Could you check a few things on this model? Use its own coordinates, in mm. A direction names the side the tool comes from. Give positions to 0.01 mm unless a question says otherwise; leave off trailing zeros. Order: outer loops, then holes, each group sorted by start corner. A loop starts at its lowest first (then second) coordinate and runs counter-clockwise, first axis right, second up. Notation, with made-up numbers: (11, -2.5) -> (41, -2.5) arc R18 cw to (41, 21.5) -> close; hole circle Ø2 at (66.25, 83.5). An arc over 180 degrees is marked (long way). Answer as CSV lines item,"result". Start each with the question number.
(1) I need wall thicknesses on L1, parallel to Y at x = -12, z = -12.55; L2, parallel to Z at x = -4, y = 2.5; L3, parallel to X at y = 10, z = -13.95. Which ranges of each line are inside material? Lowest first, please.
(2) Will these pins go through, and if not, where does the flat tip stop? pin 1 Ø5 at (x, y) = (13, 11.5) entering from +Z; pin 2 Ø5 at (y, z) = (12.5, 1) entering from -X; pin 3 Ø4.5 at (y, z) = (7.5, -6.5) entering from +X; pin 4 Ø12 at (x, z) = (0.5, -2) entering from -Y.
(3) I want a section at C-C (x = -8). Please give me the cut outline in (y, z).
(4) We'd pull the mould along X, two halves only. Please class faces 4 (the face through (11.231, 12.727, 4.728)), 5 (the face through (1, 20, -6)), 6 (the face through (0, 10, -5)): released by +X, released by -X, zero draft, split by the parting line, or undercut.
(5) I want a section at B-B (y = 10). Please give me the cut outline in (x, z).
(6) On a 3-axis mill with a long thin cutter (end or side, diameter ignored), from which of +Z, -Z, +X, -X, +Y, -Y can I reach the whole of each face in a straight line? I mean faces 1 (the face through (-9, 10, -12)), 2 (the face through (-11.642, 12.727, -13.521)), 3 (the face through (3, 10, -7)). Say none if no direction works.
(7) I want a section at D-D (z = 0.5). Please give me the cut outline in (x, y), plus the area to 3 significant figures.
(8) I want a section at A-A (x = -12). Please give me the cut outline in (y, z).
Autodesk Inventor part; units mm, degrees
ref_plane "YZ Plane" through (0, 0, 0) normal (1, 0, 0) x (0, 1, 0)
ref_plane "XZ Plane" through (0, 0, 0) normal (0, 1, 0) x (-1, 0, 0)
ref_plane "XY Plane" through (0, 0, 0) normal (0, 0, 1) x (1, 0, 0)
sketch "Sketch4" plane through (0, 0, 0) normal (0, 1, 0) x (-1, 0, 0)
  line L0 (0, 0) -> (0, -12)
  line L1 (0, -12) -> (20, -12)
  line L2 (20, -12) -> (0, -12)
  line L3 (0, -12) -> (0, -15)
  line L4 (0, -15) -> (20, -15)
  line L5 (20, -15) -> (20, -12)
  line L6 (0, 0) -> (-15.5885, 9)
  line L7 (0, 0) -> (18, 0) construction
  line L8 (-15.5885, 9) -> (0, 0)
  line L9 (0, 0) -> (-1.5, -2.5981)
  line L10 (-1.5, -2.5981) -> (-17.0885, 6.4019)
  line L11 (-17.0885, 6.4019) -> (-15.5885, 9)
  line L12 (0, 0) -> (0, -15)
  line L13 (0, -15) -> (-3, -15)
  line L14 (-3, -15) -> (-3, 0)
  line L15 (-3, 0) -> (0, 0)
  dimension "d16" = 12
  dimension "d17" = 20
  dimension "d18" = 3
  dimension "d19" = 18
  dimension "d20" = 150
  dimension "d21" = 3
  dimension "d24" = 3
extrude "Extrusion5" add sketch "Sketch4" along normal blind 20
sketch "Sketch5" plane through (3, 0, -15) normal (0, 0, -1) x (-1, 0, 0)
  line L0 (15, 0) -> (15, 10)
  circle A0 centre (15, 10) radius 2.75
  line L1 (0, 0) -> (0, 20)
  dimension "d27" = 10
  dimension "d28" = 5.5
  dimension "d36" = 15
extrude "Extrusion6" cut sketch "Sketch5" against normal blind 3
sketch "Sketch6" plane through (3, 0, -1.7321) normal (0.5, 0, -0.866) x (-0.866, 0, -0.5)
  line L0 (0, 0) -> (0, 20)
  line L1 (0, 10) -> (-10, 10)
  circle A0 centre (-10, 10) radius 2.75
  point P0 (1.7321, 0)
  dimension "d31" = 10
  dimension "d32" = 5.5
extrude "Extrusion7" cut sketch "Sketch6" against normal blind 3
fillet "Fillet1" radius 5 2 edges at (3, 10, -1.7321) (3, 10, -15)
fillet "Fillet2" radius 2 1 edges at (0, 10, -12)
properties part number "Acrylic_angle_bracket"
Final values:
1,L1,"0 to 7.25, 12.75 to 20"
1,L2,"-15 to -12"
1,L3,"-20 to -14.75, -9.25 to 1.07"
2,pin 1,"z = 8.95"
2,pin 2,"x = 0"
2,pin 3,"x = 3.01"
2,pin 4,"y = 0"
3,outline,"(0, -15) -> (20, -15) -> (20, -12) -> (0, -12) -> close"
4,face 4,"undercut"
4,face 5,"zero draft"
4,face 6,"released by -X"
5,outline,"(-20, -15) -> (-14.75, -15) -> (-14.75, -12) -> (-20, -12) -> close; (-9.25, -15) -> (-2, -15) arc R5 ccw to (3, -10) -> (3, -4.62) arc R5 cw to (5.5, -0.29) -> (9.28, 1.89) -> (7.78, 4.49) -> (0, 0) -> (0, -10) arc R2 cw to (-2, -12) -> (-9.25, -12) -> close; (12.54, 7.24) -> (14.04, 4.64) -> (17.09, 6.4) -> (15.59, 9) -> close"
6,face 1,"+Z, -X, +Y, -Y"
6,face 2,"+Z, -Z"
6,face 3,"-Z, +X, +Y, -Y"
7,outline,"(0.87, 0) -> (6.87, 0) -> (6.87, 20) -> (0.87, 20) -> close"
7,area,"120 mm²"
8,outline,"(0, -15) -> (7.25, -15) -> (7.25, -12) -> (0, -12) -> close; (12.75, -15) -> (20, -15) -> (20, -12) -> (12.75, -12) -> close"
